Source: CAD feature listing. Evaluate the final solid. Frame: model axes, mm. Round coordinates to 2 decimals unless told otherwise and drop trailing zeros. Loops run counter-clockwise (first coordinate to the right, second up) from the corner with the lowest first, then second, coordinate; pieces in that order, holes last.
(1) Section A-A, the plane x = 20.32. Return the cut outline in (y, z), plus the area to 3 significant figures.
(2) Section C-C, the plane x = 0. Return the cut outline in (y, z) (1 decimal), plus the area to 3 significant figures.
(3) First-contact query: pin 1 Ø6 at (x, z) = (62.12, 80.39) entering from +Y; pin 2 Ø2 at (x, y) = (49.5, 1) entering from +Z. Flat tips, straight axial feed; report the tip coordinate or a pass-through.
(4) Section D-D, the plane z = 59. Return the cut outline in (x, y), plus the area to 3 significant figures.
(5) Section B-B, the plane y = -0.5. Count the separate pieces of the cut face and the enclosed holes in it, plus the area to 3 significant figures.
(6) Material intervals for probe 1 along Z at (x, y) = (0, -1) (1 decimal); probe 2 along Z at (x, y) = (58, -0.1); probe 3 along X at (y, z) = (0.1, 40.64), sorted ascending.
```python
from build123d import *

# Parameters (mm, degrees)
SKETCH1_R           = 3.175
SKETCH1_R_2         = 4.8895
SKETCH1_R_3         = 1.5875
BOSS_EXTRUDE1_DEPTH = 2.4765


with BuildPart() as part:
    # Sketch1 → Boss-Extrude1 (new, symmetric)
    with BuildSketch(Plane(origin=(0, 0, 0), x_dir=(1, 0, 0), z_dir=(0, 1, 0))):
        with BuildLine():
            Line((-9.920693981, -0.985272137), (-4.645338625, -54.102765436))
            ThreePointArc((-4.645338625, -54.102765436), (13.82535886, -92.910530232), (52.781966192, -111.065199582))
            ThreePointArc((52.781966192, -111.065199582), (58.709905634, -108.665583198), (60.200009938, -102.446402065))
            ThreePointArc((60.200009938, -102.446402065), (60.977721367, -94.820202541), (66.399042003, -89.400512808))
            ThreePointArc((66.399042003, -89.400512808), (72.090603236, -80.589631254), (66.74806575, -71.56284909))
            ThreePointArc((66.74806575, -71.56284909), (51.849457493, -62.196647711), (38.60581081, -50.607856626))
            Line((38.60581081, -50.607856626), (30.607, -50.607856626))
            Line((30.607, -50.607856626), (30.607, -41.464916232))
            ThreePointArc((30.607, -41.464916232), (17.762693232, -20.754549727), (9.712854703, 2.24752837))
            ThreePointArc((9.712854703, 2.24752837), (-1.619737346, 9.837041282), (-9.920693981, -0.985272137))
        make_face()
        Circle(SKETCH1_R, mode=Mode.SUBTRACT)
        with Locations((62.123011123, -80.394598631)):
            Circle(SKETCH1_R_2, mode=Mode.SUBTRACT)
        with Locations((54.567235003, -104.644758367)):
            Circle(SKETCH1_R, mode=Mode.SUBTRACT)
        with Locations((10.16, -40.64)):
            Circle(SKETCH1_R_3, mode=Mode.SUBTRACT)
        with Locations((20.32, -81.28)):
            Circle(SKETCH1_R_3, mode=Mode.SUBTRACT)
    extrude(amount=BOSS_EXTRUDE1_DEPTH, both=True)


solid = part.part
```
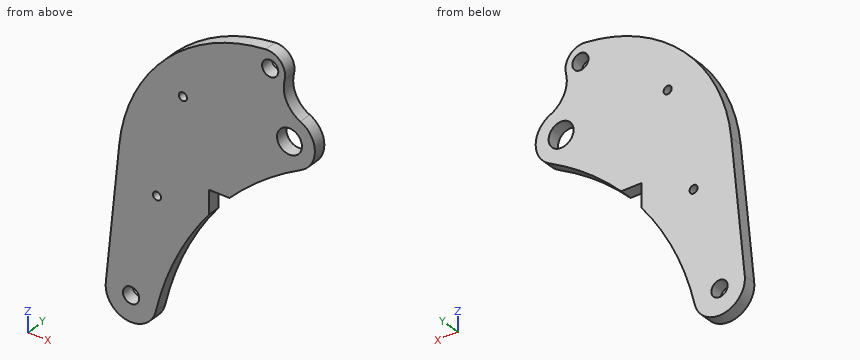
Output values:
1. outline: (-2.48, 25.78) - (2.48, 25.78) - (2.48, 79.69) - (-2.48, 79.69) - close; (-2.48, 82.87) - (2.48, 82.87) - (2.48, 98.53) - (-2.48, 98.53) - close
1. area: 345 mm2
2. outline: (-2.5, -10) - (2.5, -10) - (2.5, -3.2) - (-2.5, -3.2) - close; (-2.5, 3.2) - (2.5, 3.2) - (2.5, 72.4) - (-2.5, 72.4) - close
2. area: 377 mm2
3. pin 1: passes through
3. pin 2: stops at z = 110.82
4. outline: (-3.97, -2.48) - (47.76, -2.48) - (47.76, 2.48) - (-3.97, 2.48) - close
4. area: 256 mm2
5. separate pieces: 1
5. enclosed holes: 5
5. area: 4,520 mm2
6. probe 1: z = -10 to -3.2, 3.2 to 72.4
6. probe 2: z = 66.46 to 77.77, 83.02 to 109.38
6. probe 3: x = -5.98 to 8.57, 11.75 to 29.97
